Verification items for the finished model (mm, model axes). Face numbers are marked on the shaded views. A direction names the side the tool comes from. Give positions to 0.01 mm unless a question says otherwise; leave off trailing zeros. Order: outer loops, then holes, each group sorted by start corner. A loop starts at its lowest first (then second) coordinate and runs counter-clockwise, first axis right, second up.
(1) Mould release check, pull along Y, two halves, no side actions. Record for the marked faces 6, 7 and 8: pulls with the +Y half, pulls with the -Y half, needs draft (parallel to the pull), parting line crosses it, or undercut.
(2) Scan lines: L1, parallel to Y at x = 21, z = -4; L2, parallel to Y at x = 12.5, z = 7; L3, parallel to X at y = 23.5, z = -29.5. Record each from-to range of solid material in increasing order.
(3) Sectioned sample at C-C on y = 33. Record the cut outline in (x, z), plus the area to 3 significant figures.
(4) Sectioned sample at B-B on x = 30. Record the cut outline in (y, z).
(5) Gauge pin test, flat ends, axial feed: pin 1 (22 mm diameter, centred on x = 10, z = 7.5, fed in from +Y); pin 2 (6 mm diameter, centred on y = 62, z = -10, fed in from +X); pin 3 (8 mm diameter, centred on y = 10, z = -28, fed in from +X); pin 4 (6 mm diameter, centred on x = 13.5, z = -51, fed in from +Y). Record the tip position at first contact, or that the pin passes through.
(6) Access from +Z, -Z, +X, -X, +Y, -Y to the whole of each face (thin tool, end or side, straight path). Record for the marked faces 1, 2, 3, 4 and 5.
(7) Sectioned sample at A-A on z = -16.5. Record the cut outline in (x, y).
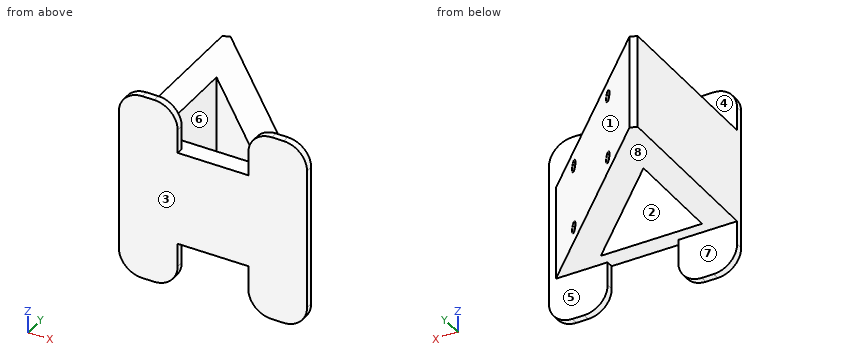
Autodesk Inventor part; units mm, degrees
ref_plane "YZ Plane" through (0, 0, 0) normal (1, 0, 0) x (0, 1, 0)
ref_plane "XZ Plane" through (0, 0, 0) normal (0, 1, 0) x (-1, 0, 0)
ref_plane "XY Plane" through (0, 0, 0) normal (0, 0, 1) x (1, 0, 0)
sketch "Sketch1" plane through (0, 0, 0) normal (0, 0, 1) x (1, 0, 0)
  line L0 (0, 0) -> (80, 0)
  line L1 (80, 0) -> (80, 80)
  line L2 (80, 80) -> (0, 80)
  line L3 (0, 80) -> (0, 0)
  line L4 (80, 0) -> (0, 80)
  dimension "d0" = 80
  dimension "d1" = 80
  dimension "d2" = 45
extrude "Extrusion1" add sketch "Sketch1" against normal blind 40 contours L3 L4 L0
sketch "Sketch2" plane through (80, 0, -40) normal (0.7071, 0.7071, 0) x (-0.7071, 0.7071, 0)
  circle A0 centre (78.1371, 33.5) radius 2.1
  circle A1 centre (78.1371, 6.5) radius 2.1
  line L0 (0, 40) -> (113.1371, 40)
  line L1 (113.1371, 0) -> (0, 0)
  circle A2 centre (29.6371, 33.5) radius 2.1
  circle A3 centre (29.6371, 6.5) radius 2.1
  line L2 (113.1371, 40) -> (113.1371, 0)
  point P0 (56.5685, 40)
  dimension "d5" = 27
  dimension "d6" = 4.2
  dimension "d7" = 4.2
  dimension "d8" = 6.5
  dimension "d10" = 27
  dimension "d11" = 4.2
  dimension "d12" = 4.2
  dimension "d13" = 48.5
  dimension "d29" = 35
  dimension "d30" = 35
  dimension "d31" = 48.5
  dimension "d32" = 6.5
extrude "Extrusion2" cut sketch "Sketch2" against normal blind 10
fillet "Fillet1" radius 0.4 4 edges at (26.2337, 53.7663, -33.5) (26.2337, 53.7663, -6.5) (60.5283, 19.4717, -6.5) (60.5283, 19.4717, -33.5)
sketch "Sketch3" plane through (0, 0, -40) normal (0, 0, -1) x (-1, 0, 0)
  line L0 (0, 80) -> (-80, 0)
  line L1 (0, 0) -> (0, 80)
  line L2 (-80, 0) -> (0, 80)
  line L3 (0, 80) -> (0, 0)
  line L4 (0, 0) -> (-80, 0)
  line L5 (-91.5147, -28.4853) -> (-12, 51.0294)
  line L6 (-12, 51.0294) -> (-12, 0)
  line L7 (-12, 8) -> (-55.0294, 8)
  dimension "d17" = 12
  dimension "d18" = 8
extrude "Extrusion3" cut sketch "Sketch3" against normal blind 40 contours L5 L6 L7
sketch "Sketch4" plane through (0, 0, 0) normal (0, -1, 0) x (1, 0, 0)
  line L0 (-20, -60) -> (80, -60)
  line L1 (80, -60) -> (80, 20)
  line L2 (80, 20) -> (-20, 20)
  line L3 (-20, 20) -> (-20, -60)
  line L4 (80, 0) -> (80, -40)
  line L5 (80, -40) -> (0, -40)
  line L6 (0, 0) -> (80, 0)
  line L7 (50, 20) -> (10, 20)
  line L8 (10, 20) -> (10, -60)
  line L9 (10, -60) -> (50, -60)
  line L10 (50, -60) -> (50, 20)
  point P0 (10, 0)
  point P1 (10, 20)
  point P2 (10, -40)
  point P3 (50, -40)
  point P4 (50, 0)
  dimension "d21" = 100
  dimension "d22" = 0
  dimension "d23" = 20
  dimension "d24" = 20
  dimension "d25" = 30
  dimension "d26" = 30
extrude "Extrusion4" [suppressed]
chamfer "Chamfer1" distance 4 angle 45 1 edges at (0, 80, -20)
fillet "Fillet2" [suppressed]
sketch "Sketch5" plane through (0, 0, 0) normal (0, -1, 0) x (1, 0, 0)
  line L0 (0, 20) -> (80, 20)
  line L1 (80, 20) -> (80, -60)
  line L2 (80, -60) -> (0, -60)
  line L3 (0, -60) -> (0, 20)
  line L4 (0, 0) -> (80, 0)
  line L5 (80, -40) -> (0, -40)
  line L6 (80, 0) -> (80, -40)
  line L7 (25, 20) -> (55, 20)
  line L8 (55, 20) -> (55, -60)
  line L9 (55, -60) -> (25, -60)
  line L10 (25, -60) -> (25, 20)
  dimension "d37" = 20
  dimension "d38" = 20
  dimension "d39" = 0
  dimension "d40" = 80
  dimension "d41" = 25
  dimension "d42" = 25
extrude "Extrusion5" add sketch "Sketch5" against normal blind 3 contours L0 L10 L4 L3 | L4 L10 L5 L3 | L0 L1 L4 L8 | L5 L10 L2 L3 | L4 L1 L5 L8 | L5 L1 L2 L8
fillet "Fillet3" radius 10 8 edges at (25, 1.5, 20) (0, 1.5, 20) (55, 1.5, 20) (80, 1.5, 20) (80, 1.5, -60) (55, 1.5, -60) (25, 1.5, -60) (0, 1.5, -60)
properties part number "Gravitational viscometer P2"
Ans:
1. face 6: undercut
1. face 7: pulls with the +Y half
1. face 8: needs draft
2. L1: y = 0 to 8, 42.03 to 59
2. L2: y = 0 to 3
2. L3: x = 0 to 12, 39.53 to 56.5
3. outline: (0, -40) - (12, -40) - (12, 0) - (0, 0) - close; (30.03, -40) - (47, -40) - (47, 0) - (30.03, 0) - close
3. area: 1,160 mm2
4. outline: (0, -40) - (8, -40) - (8, 0) - (0, 0) - close; (33.03, -40) - (50, -40) - (50, 0) - (33.03, 0) - close
5. pin 1: stops at y = 77.17
5. pin 2: stops at x = 21
5. pin 3: stops at x = 74
5. pin 4: stops at y = 3
6. face 1: +Z, -Z, +X, +Y
6. face 2: +Z, -Z
6. face 3: +Z, -Z, +X, -X, -Y
6. face 4: +Z, +X, -X, +Y
6. face 5: +X, +Y
7. outline: (0, 0) - (80, 0) - (80, 3) - (77, 3) - (2.83, 77.17) - (0, 76) - close; hole (12, 8) - (55.03, 8) - (12, 51.03) - close
